Model file for the job. Use its own axes, mm. Face numbers are marked on the shaded views. Coordinates: 2 decimals unless noted, no trailing zeros. Order: outer loops, then holes, each group sorted by start corner. A loop starts at its lowest first (then second) coordinate and runs counter-clockwise, first axis right, second up. Notation, with made-up numbers: (42, 62.5) - (63, 62.5) arc R12 cw to (63, 82.5) - close; hole circle Ø1 at (-23, 75). An arc over 180 degrees is marked (long way). Put each result on its own line as item: value. Start each with the question number.
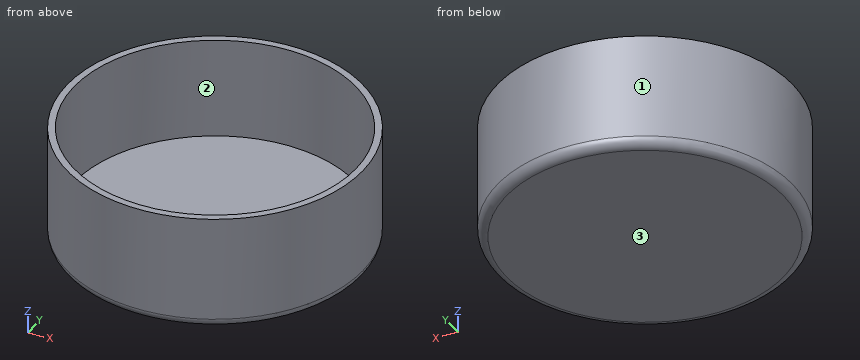
```python
from build123d import *

# Parameters (mm, degrees)
F0_R     = 32.25
F0_R_2   = 30.75
F1_DEPTH = 22
F2_R     = 32.25
F3_DEPTH = 3
F4_R     = 2


with BuildPart() as f1:
    # F0 (on Top) → F1 (new body)
    with BuildSketch(Plane.XY):
        Circle(F0_R)
        Circle(F0_R_2, mode=Mode.SUBTRACT)
    extrude(amount=F1_DEPTH)

    # F2 (on Top) → F3 (join)
    with BuildSketch(Plane.XY):
        Circle(F2_R)
    extrude(amount=-F3_DEPTH)

    # F4
    f4_edges = [f1.edges().sort_by_distance(p)[0] for p in [
        (-32.25, 0, -3),
    ]]
    fillet(f4_edges, radius=F4_R)


solid = f1.part
```
Item 1: Slice it at A-A, the plane x = 0. Give the cut face in (y, z).
Item 2: Wall check: line 1 along Y through (x, z) = (0, 7.5); line 2 along X through (y, z) = (-1, 7); line 3 along Z through (x, y) = (8, 23). Give the ranges that are in metal, low to high.
Item 3: Slice it at C-C, the plane z = 17.5. Give the cut face in (x, y), plus the area to 3 significant figures.
Item 4: Flat gauge pins, fed straight in: pin 1 Ø12 at (y, z) = (-20, 2.5) entering from -X; pin 2 Ø5 at (y, z) = (-9, 12) entering from +X; pin 3 Ø18.5 at (x, y) = (12, -13) entering from +Z. Where does each tip first touch, or does it go through?
Item 5: Pull direction Y, two halves, no side cores. Call the marked faces 1, 2 and 3: pulls with the +Y half, pulls with the -Y half, needs draft (parallel to the pull), parting line crosses it, or undercut.
Here are the results:
1. outline: (-32.25, -1) arc R2 ccw to (-30.25, -3) - (30.25, -3) arc R2 ccw to (32.25, -1) - (32.25, 22) - (30.75, 22) - (30.75, 0) - (-30.75, 0) - (-30.75, 22) - (-32.25, 22) - close
2. line 1: y = -32.25 to -30.75, 30.75 to 32.25
2. line 2: x = -32.23 to -30.73, 30.73 to 32.23
2. line 3: z = -3 to 0
3. outline: circle Ø64.5 at (0, 0); hole circle Ø61.5 at (0, 0)
3. area: 297 mm^2
4. pin 1: stops at x = -29.05
4. pin 2: stops at x = 31.59
4. pin 3: stops at z = 0
5. face 1: parting line crosses it
5. face 2: undercut
5. face 3: needs draft
